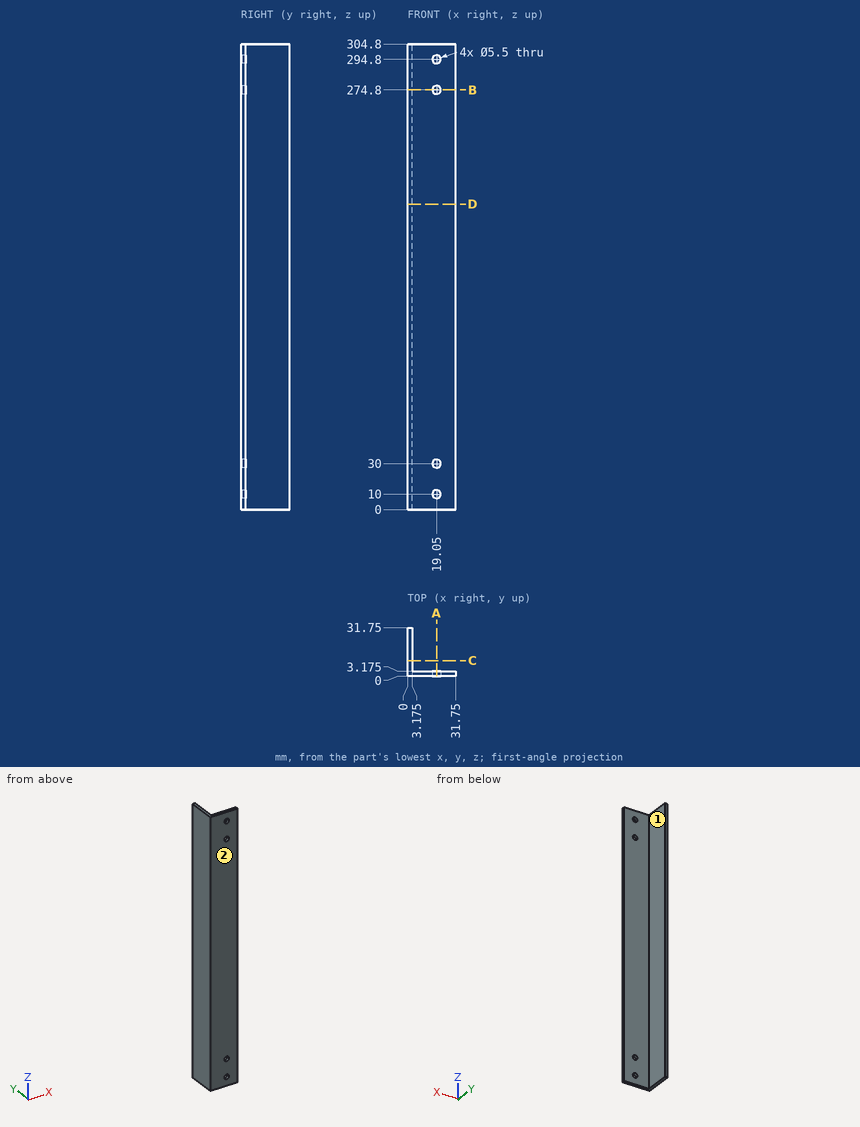
Geometry check sheet. Reference: drawing and pictorial views, mm from the part's lowest x, y, z. A direction names the side the tool comes from. Round coordinates to 2 decimals unless told otherwise and drop trailing zeros. Order: outer loops, then holes, each group sorted by start corner. A loop starts at its lowest first (then second) coordinate and runs counter-clockwise, first axis right, second up. Notation, with made-up numbers: (60, 24.5) -> (93, 24.5) arc R14 cw to (93, 32.5) -> close; hole circle Ø9 at (66, 9.25). An arc over 180 degrees is marked (long way). One line per item, written item: value. Start each with the question number.
Q1. Gauge pin test, flat ends, axial feed: pin 1 Ø5 at (y, z) = (13.5, 152.5) entering from -X; pin 2 Ø8.5 at (y, z) = (21, 192.5) entering from +X (3 decimals); pin 3 Ø8.5 at (x, z) = (17, 151.5) entering from +Y (3 decimals). Record the tip position at first contact, or that the pin passes through.
Q2. Cross-section at B-B (z = 274.8). Record the boundary of the cut face in (x, y) (3 decimals), and give its area (3 significant figures).
Q3. Set-up check for the marked faces 1 and 2: record each of +Z, -Z, +X, -X, +Y, -Y from which the full face is reachable in a straight line by a thin tool's end or side.
Q4. Cross-section at D-D (z = 200). Record the boundary of the cut face in (x, y) (3 decimals), and give its area (3 significant figures).
Q5. Cross-section at C-C (y = 10). Record the boundary of the cut face in (x, z) (3 decimals), and give its area (3 significant figures).
Q6. Thickness scan on line 1 (Z direction, x = 19, y = 2); line 2 (X direction, y = 1.35, z = 274.8); line 3 (Y direction, x = 12, z = 261.5) (3 decimals). Record the ranges inside material, lowest first.
Q7. Cross-section at A-A (x = 19.05). Record the boundary of the cut face in (y, z) (3 decimals), and give its area (3 significant figures).
Completed:
1. pin 1: stops at x = 0
1. pin 2: stops at x = 3.175
1. pin 3: stops at y = 3.175
2. outline: (0, 0) -> (16.3, 0) -> (16.3, 3.175) -> (3.175, 3.175) -> (3.175, 31.75) -> (0, 31.75) -> close; (21.8, 0) -> (31.75, 0) -> (31.75, 3.175) -> (21.8, 3.175) -> close
2. area: 174 mm²
3. face 1: +Z, -Z, +X, +Y
3. face 2: +Z, -Z, +X, -X, -Y
4. outline: (0, 0) -> (31.75, 0) -> (31.75, 3.175) -> (3.175, 3.175) -> (3.175, 31.75) -> (0, 31.75) -> close
4. area: 192 mm²
5. outline: (0, 0) -> (3.175, 0) -> (3.175, 304.8) -> (0, 304.8) -> close
5. area: 968 mm²
6. line 1: z = 0 to 7.25, 12.75 to 27.25, 32.75 to 272.05, 277.55 to 292.05, 297.55 to 304.8
6. line 2: x = 0 to 16.3, 21.8 to 31.75
6. line 3: y = 0 to 3.175
7. outline: (0, 0) -> (3.175, 0) -> (3.175, 7.25) -> (0, 7.25) -> close; (0, 12.75) -> (3.175, 12.75) -> (3.175, 27.25) -> (0, 27.25) -> close; (0, 32.75) -> (3.175, 32.75) -> (3.175, 272.05) -> (0, 272.05) -> close; (0, 277.55) -> (3.175, 277.55) -> (3.175, 292.05) -> (0, 292.05) -> close; (0, 297.55) -> (3.175, 297.55) -> (3.175, 304.8) -> (0, 304.8) -> close
7. area: 898 mm²
